For this review, take the finished solid that the model builds, in its own axes (mm). A direction names the side the tool comes from. Coordinates: 2 decimals unless noted, no trailing zeros. Loops run counter-clockwise (first coordinate to the right, second up) from the corner with the lowest first, then second, coordinate; pieces in that order, holes last. Notation, with made-up numbers: (-34.75, 87) - (-10.75, 87) arc R14 ccw to (-10.75, 95) - close; hole circle Ø9 at (-24.5, 68.25). An arc over 180 degrees is marked (long way). Answer as a JSON object with one key per item and string values. Group by question number.
Item 1: Clearance check with flat-ended pins moving along their axes: pin 1 (5 mm diameter, centred on x = 0.5, z = 18, fed in from +Y); pin 2 (3 mm diameter, centred on x = 3.5, z = 35, fed in from +Y); pin 3 (3 mm diameter, centred on x = 3.35, z = 34.85, fed in from -Y). State where each tip first meets the part, or that it passes through.
Item 2: We need section C-C (x = -1). Give the boundary of the cut face in (y, z), then the cut area to 3 significant figures.
Item 3: To check wall thickness, follow line 1 (X direction, y = 7.25, z = 9); line 2 (X direction, y = 7.5, z = -8); line 3 (Y direction, x = 3, z = 13). State the ranges of each line that lie inside material, in increasing order.
Item 4: Mouldability with a two-part tool opening along Z and no side actions: class faces 5 (the cylindrical face through (11.92, 8.46, -30.78)), 6 (the flat face through (22.5, 7, 1)) as released by +Z, released by -Z, zero draft, split by the parting line, or undercut.
Item 5: Tool access review of faces 1 (the flat face through (20.4, 9.601, -1.1)), 2 (the cylindrical face through (2.973, 1.479, 33.142)), 3 (the cylindrical face through (-13.99, 8.46, 30.73)), 4 (the flat face through (17, 5, -1.435)): name each direction out of +Z, -Z, +X, -X, +Y, -Y from which nothing blocks a thin tool from reaching the whole face with its end or side.
Item 6: We need section B-B (y = 8.5). Give the boundary of the cut face in (x, z) (3 decimals).
Item 7: We need section A-A (y = 12). Give the boundary of the cut face in (x, z), then the cut area to 3 significant figures.
Item 8: We need section D-D (z = 11). Give the boundary of the cut face in (x, y), then the cut area to 3 significant figures.
from build123d import *

# Parameters (mm, degrees)
CROQUIS1_W              = 45
CROQUIS1_H              = 75
SALIENTE_EXTRUIR1_DEPTH = 11
CROQUIS2_W              = 30
CROQUIS2_H              = 64
CORTAR_EXTRUIR1_DEPTH   = 7
CROQUIS3_W              = 5
CROQUIS3_H              = 3.7
SALIENTE_EXTRUIR2_DEPTH = 2
CROQUIS4_R              = 1.14
SALIENTE_EXTRUIR3_DEPTH = 5
CROQUIS8_W              = 5.042710394
CROQUIS8_H              = 23.757603043
CORTAR_EXTRUIR2_DEPTH   = 12
CROQUIS10_W             = 6.704370917
CROQUIS10_H             = 75
CORTAR_EXTRUIR3_DEPTH   = 18
CROQUIS11_W             = 11.359484983
CROQUIS11_H             = 5.310310124
CROQUIS11_W_2           = 4.5
CROQUIS11_H_2           = 3.836618742
CORTAR_EXTRUIR4_DEPTH   = 1
CROQUIS13_W             = 10
CROQUIS13_H             = 1.398702395
CROQUIS13_W_2           = 3.73
CROQUIS13_H_2           = 1.377461041
CORTAR_EXTRUIR5_DEPTH   = 38.3
CROQUIS15_R             = 1.75
CORTAR_EXTRUIR7_DEPTH   = 3
CROQUIS16_W             = 19.147118229
CROQUIS16_H             = 6.405137331
CORTAR_EXTRUIR8_DEPTH   = 10
CROQUIS17_W             = 0.795629083
CROQUIS17_H             = 4.286046827
CROQUIS17_H_2           = 3.741316105
SALIENTE_EXTRUIR4_DEPTH = 3
CROQUIS18_R             = 1.75
CORTAR_EXTRUIR9_DEPTH   = 3


with BuildPart() as part:
    # Croquis1 → Saliente-Extruir1 (new body)
    with BuildSketch(Plane(origin=(0, 0, 0), x_dir=(1, 0, 0), z_dir=(0, 1, 0))):
        Rectangle(CROQUIS1_W, CROQUIS1_H)
    extrude(amount=SALIENTE_EXTRUIR1_DEPTH)

    # Croquis2 → Cortar-Extruir1 (cut)
    with BuildSketch(Plane(origin=(0, 11, 0), x_dir=(1, 0, 0), z_dir=(0, 1, 0))):
        Rectangle(CROQUIS2_W, CROQUIS2_H)
    extrude(amount=-CORTAR_EXTRUIR1_DEPTH, mode=Mode.SUBTRACT)

    # Croquis3 → Saliente-Extruir2 (add)
    with BuildSketch(Plane(origin=(0, 4, 0), x_dir=(1, 0, 0), z_dir=(0, 1, 0))):
        with Locations((12.5, -30.15)):
            Rectangle(CROQUIS3_W, CROQUIS3_H)
        with Locations((-12.5, -30.15)):
            Rectangle(CROQUIS3_W, CROQUIS3_H)
        with Locations((12.5, 30.15)):
            Rectangle(CROQUIS3_W, CROQUIS3_H)
        with Locations((-12.5, 30.15)):
            Rectangle(CROQUIS3_W, CROQUIS3_H)
    extrude(amount=SALIENTE_EXTRUIR2_DEPTH)

    # Croquis4 → Saliente-Extruir3 (add)
    with BuildSketch(Plane(origin=(0, 6, 0), x_dir=(1, 0, 0), z_dir=(0, 1, 0))):
        with Locations((-13.085, -30.04)):
            Circle(CROQUIS4_R)
        with Locations((12.065, -30.04)):
            Circle(CROQUIS4_R)
        with Locations((-13.085, 29.65)):
            Circle(CROQUIS4_R)
        with Locations((12.065, 29.65)):
            Circle(CROQUIS4_R)
    extrude(amount=SALIENTE_EXTRUIR3_DEPTH)

    # Croquis8 → Cortar-Extruir2 (cut)
    with BuildSketch(Plane(origin=(0, 11, 0), x_dir=(1, 0, 0), z_dir=(0, 1, 0))):
        with Locations((17.521355197, -10.443778519)):
            Rectangle(CROQUIS8_W, CROQUIS8_H)
    extrude(amount=-CORTAR_EXTRUIR2_DEPTH, mode=Mode.SUBTRACT)

    # Croquis10 → Cortar-Extruir3 (cut)
    with BuildSketch(Plane(origin=(0, 11, 0), x_dir=(1, 0, 0), z_dir=(0, 1, 0))):
        with Locations((-19.147814542, 0)):
            Rectangle(CROQUIS10_W, CROQUIS10_H)
    extrude(amount=-CORTAR_EXTRUIR3_DEPTH, mode=Mode.SUBTRACT)

    # Croquis11 → Cortar-Extruir4 (cut)
    with BuildSketch(Plane.ZY.offset(15.795629083)):
        with Locations((23.268650218, 8.344844938)):
            Rectangle(CROQUIS11_W, CROQUIS11_H)
        with Locations((11.597591621, 9.081690629)):
            Rectangle(CROQUIS11_W_2, CROQUIS11_H_2)
    extrude(amount=-CORTAR_EXTRUIR4_DEPTH, mode=Mode.SUBTRACT)

    # Croquis13 → Cortar-Extruir5 (cut)
    with BuildSketch(Plane.ZY.offset(15.795629083)):
        with Locations((0.061544794, 10.300648802)):
            Rectangle(CROQUIS13_W, CROQUIS13_H)
        with Locations((-5.073455206, 10.311269479)):
            Rectangle(CROQUIS13_W_2, CROQUIS13_H_2)
    extrude(amount=-CORTAR_EXTRUIR5_DEPTH, mode=Mode.SUBTRACT)

    # Croquis15 → Cortar-Extruir7 (cut)
    with BuildSketch(Plane.XZ):
        with Locations((3.352185458, -34.85)):
            Circle(CROQUIS15_R)
        with Locations((3.352185458, 34.85)):
            Circle(CROQUIS15_R)
    extrude(amount=-CORTAR_EXTRUIR7_DEPTH, mode=Mode.SUBTRACT)

    # Croquis16 → Cortar-Extruir8 (cut)
    with BuildSketch(Plane(origin=(0, 0, -37.5), x_dir=(-1, 0, 0), z_dir=(0, 0, -1))):
        with Locations((0.122687914, 7.582003397)):
            Rectangle(CROQUIS16_W, CROQUIS16_H)
    extrude(amount=-CORTAR_EXTRUIR8_DEPTH, mode=Mode.SUBTRACT)

    # Croquis17 → Saliente-Extruir4 (add)
    with BuildSketch(Plane(origin=(0, 11, 0), x_dir=(1, 0, 0), z_dir=(0, 1, 0))):
        Polygon((-15.795629083, 6.938455206), (-15, 6.938455206), (-15, 32), (15, 32), (15, 6.938455206), (22.5, 6.938455206), (22.5, 37.5), (-15.795629083, 37.5), align=None)
        with Locations((-15.397814542, -7.204568208)):
            Rectangle(CROQUIS17_W, CROQUIS17_H)
        with Locations((-15.397814542, -15.718249674)):
            Rectangle(CROQUIS17_W, CROQUIS17_H_2)
        Polygon((22.5, -5.061544794), (20.042710394, -5.061544794), (20.042710394, -22.32258004), (15, -22.32258004), (15, -32), (-15, -32), (-15, -28.948392709), (-15.795629083, -28.948392709), (-15.795629083, -37.5), (22.5, -37.5), align=None)
    extrude(amount=SALIENTE_EXTRUIR4_DEPTH)

    # Croquis18 → Cortar-Extruir9 (cut)
    with BuildSketch(Plane(origin=(0, 14, 0), x_dir=(1, 0, 0), z_dir=(0, 1, 0))):
        with Locations((3.352185458, -34.85)):
            Circle(CROQUIS18_R)
        with Locations((3.352185458, 34.85)):
            Circle(CROQUIS18_R)
    extrude(amount=-CORTAR_EXTRUIR9_DEPTH, mode=Mode.SUBTRACT)


solid = part.part
Check sheet entries:
{
 "1": {"pin 1": "stops at y = 4", "pin 2": "stops at y = 11", "pin 3": "stops at y = 3"},
 "2": {"outline": "(0, -37.5) - (4.38, -37.5) - (4.38, -32) - (4, -32) - (4, 32) - (14, 32) - (14, 37.5) - (0, 37.5) - close; (10.78, -37.5) - (14, -37.5) - (14, -32) - (10.78, -32) - close", "area": "375 mm2"},
 "3": {"line 1": "x = -15.8 to -15, 20.04 to 22.5", "line 2": "x = -15.8 to -15, 15 to 22.5", "line 3": "y = 0 to 4"},
 "4": {"face 5": "undercut", "face 6": "zero draft"},
 "5": {"face 1": "+X, -X, +Y", "face 2": "-Y", "face 3": "+Y", "face 4": "+Y, -Y"},
 "6": {"outline": "(-15.796, -37.5) - (-9.696, -37.5) - (-9.696, -32) - (-15, -32) - (-15, 9.348) - (-15.796, 9.348) - close; (-15.796, 13.848) - (-15, 13.848) - (-15, 17.589) - (-15.796, 17.589) - close; (-15.796, 28.948) - (-15, 28.948) - (-15, 32) - (15, 32) - (15, 22.323) - (20.043, 22.323) - (20.043, -1.435) - (15, -1.435) - (15, -32) - (9.451, -32) - (9.451, -37.5) - (22.5, -37.5) - (22.5, 37.5) - (-15.796, 37.5) - close; circle Ø2.28 at (-13.085, -29.65); circle Ø2.28 at (-13.085, 30.04); circle Ø2.28 at (12.065, -29.65); circle Ø2.28 at (12.065, 30.04)"},
 "7": {"outline": "(-15.8, -37.5) - (22.5, -37.5) - (22.5, -6.94) - (15, -6.94) - (15, -32) - (-15, -32) - (-15, -6.94) - (-15.8, -6.94) - close; (-15.8, 5.06) - (-15, 5.06) - (-15, 9.35) - (-15.8, 9.35) - close; (-15.8, 13.85) - (-15, 13.85) - (-15, 17.59) - (-15.8, 17.59) - close; (-15.8, 28.95) - (-15, 28.95) - (-15, 32) - (15, 32) - (15, 22.32) - (20.04, 22.32) - (20.04, 5.06) - (22.5, 5.06) - (22.5, 37.5) - (-15.8, 37.5) - close; hole circle Ø3.5 at (3.35, -34.85); hole circle Ø3.5 at (3.35, 34.85)", "area": "734 mm2"},
 "8": {"outline": "(-15.8, 0) - (15, 0) - (15, 4) - (-15, 4) - (-15, 7.16) - (-15.8, 7.16) - close; (20.04, 0) - (22.5, 0) - (22.5, 14) - (20.04, 14) - close", "area": "160 mm2"}
}
